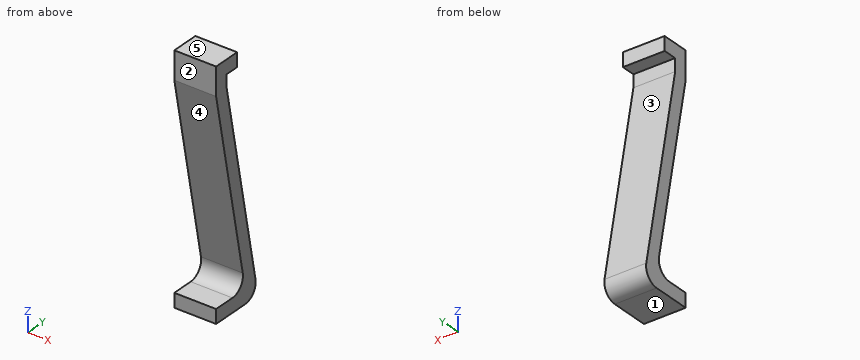
```python
from build123d import *

# Parameters (mm, degrees)
SALIENTE_EXTRUIR1_DEPTH = 30


with BuildPart() as part:
    # Croquis2 → Saliente-Extruir1 (new body)
    with BuildSketch(Plane(origin=(0, 0, 0), x_dir=(0, 0, -1), z_dir=(1, 0, 0))):
        with BuildLine():
            Line((-102.260641265, 0), (-82.307345408, 0))
            Line((-82.307345408, 0), (47.828906849, 25.352631084))
            ThreePointArc((47.828906849, 25.352631084), (56.100280199, 23.254742154), (59.741117951, 15.537161217))
            Line((59.741117951, 15.537161217), (59.741117951, 0))
            Line((59.741117951, 0), (69.741117951, 0))
            Line((69.741117951, 0), (69.741117951, 27.673321039))
            ThreePointArc((69.741117951, 27.673321039), (66.100280199, 35.390901976), (57.828906849, 37.488790906))
            Line((57.828906849, 37.488790906), (-83.272354624, 10))
            Line((-83.272354624, 10), (-92.283993337, 10))
            Line((-92.283993337, 10), (-92.283993337, 20))
            Line((-92.283993337, 20), (-102.260641265, 20))
            Line((-102.260641265, 20), (-102.260641265, 0))
        make_face()
    extrude(amount=SALIENTE_EXTRUIR1_DEPTH)


solid = part.part
```
The listing builds one solid part. Answer for the finished solid, in the listing's coordinates (mm). Face numbers are marked on the shaded views. A direction names the side the tool comes from. Give positions to 0.01 mm unless a question says otherwise; leave off trailing zeros. Write each loop counter-clockwise with the first axis right and the second up, starting at its lowest first coordinate (ties: lowest second). Pieces come first, ordered by that corner, then holes. Notation, with made-up numbers: M 51,39 L 95,39 A17 cw 95,44 Z; hole C 40.5,58.25 d5. An arc over 180 degrees is marked long. Write each question's results on one line, items separated by ' | '.
Q1. For a pull along Z with two mould halves and no side action, classify the marked faces 1, 2 and 3 as released by +Z, released by -Z, zero draft, split by the parting line, or undercut.
Output values:
face 1: released by -Z | face 2: zero draft | face 3: undercut
Q2. A tool of negligible diameter and unlimited length cuts with its end or side. For the marked faces 4 and 5, from which of +Z, -Z, +X, -X, +Y, -Y can it reach the whole face along a straight path? Write none if from no direction.
Output values:
face 4: +X, -X, -Y | face 5: +Z, +X, -X, +Y, -Y
Q3. Flat-ended cylindrical pins translate along their axes: P1, Ø10, axis at y = 9, z = 60, coming from the -X side; P2, Ø7, axis at x = 14.5, z = 88.5, coming from the +Y side; P3, Ø5, axis at x = 11, z = 98, coming from the +Y side; P4, Ø2, axis at y = 12.5, z = 10, coming from the +X side. Find the tip coordinate at first contact, or state that the pin passes through.
Output values:
P1: x = 0 | P2: y = 10 | P3: y = 20 | P4: through
Q4. Consider L1, parallel to Y at x = 28.5, z = 88; L2, parallel to Y at x = 23, z = -32.5. Determine where each line is inside the solid, lowest interval first. Write a range as from..to.
Output values:
L1: 0..10 | L2: 22.37..32.55
Q5. Section C-C, the plane z = -22 is taken. Write down the section's boundary in (x, y), then the cut area to 3 significant figures.
Output values:
outline: M 0,20.32 L 30,20.32 L 30,30.51 L 0,30.51 Z | area: 306 mm2
Q6. Section B-B, the plane y = 7.5 is taken. Write down the section's boundary in (x, z), then the cut area to 3 significant figures.
Output values:
outline: M 0,-69.74 L 30,-69.74 L 30,-59.74 L 0,-59.74 Z; M 0,43.81 L 30,43.81 L 30,102.26 L 0,102.26 Z | area: 2,050 mm2
Q7. Section A-A, the plane x = 24.5 is taken. Write down the section's boundary in (y, z).
Output values:
outline: M 0,-69.74 L 27.67,-69.74 A10 ccw 37.49,-57.83 L 10,83.27 L 10,92.28 L 20,92.28 L 20,102.26 L 0,102.26 L 0,82.31 L 25.35,-47.83 A10 cw 15.54,-59.74 L 0,-59.74 Z
Q8. Section D-D, the plane y = 30 is taken. Write down the section's boundary in (x, z), then the cut area to 3 significant figures.
Output values:
outline: M 0,-69.47 L 30,-69.47 L 30,-19.39 L 0,-19.39 Z | area: 1,500 mm2
